Verification items for the finished model (mm, model axes). A direction names the side the tool comes from. Coordinates: 2 decimals unless noted, no trailing zeros. Write each loop counter-clockwise with the first axis right and the second up, starting at its lowest first coordinate (ties: lowest second). Pieces come first, ordered by that corner, then holes. Notation, with made-up numbers: (4.25, -14) - (48.25, -14) arc R22 cw to (48.25, 11) - close; hole circle Ø8 at (47, 0.25). An arc over 180 degrees is marked (long way). Use one line per item in the form item = value. Start each with the question number.
(1) Sectioned sample at B-B (y = -6). Record the cut outline in (x, z) (3 decimals), and give its area (3 significant figures).
(2) Mould release check, pull along Z, two halves, no side actions. Record for faces 1 (the cylindrical face through (-1.57, -12.4, 2.75)), 2 (the flat face through (-1.57, -1.99, 78.3)), 3 (the cylindrical face through (-1.565, -37.718, -5.774)): released by +Z, released by -Z, zero draft, split by the parting line, or undercut.
(3) Gauge pin test, flat end, axial feed: pin 1 Ø1.5 at (x, z) = (-2.5, 69) entering from +Y. Record the tip position at first contact, or that the pin passes through.
(4) Material ranges on line 1 (Y direction, x = -1.25, z = 31.75) (3 decimals); line 2 (Y direction, x = -1.85, z = 2) (3 decimals); line 3 (Y direction, x = -1.85, z = 0), recorded low to high. Write a range as [from, to].
(5) Sectioned sample at C-C (x = -2.4). Count the separate pieces of the cut face and the enclosed holes in it, and give its area (3 significant figures).
(6) Tool access check on faces 4 (the flat face through (-1.565, -38.704, 43.485)), 5 (the cylindrical face through (-1.57, 35.54, 2.3)), 6 (the cylindrical face through (-1.57, 29.59, 41.58)). Record the directions out of +Z, -Z, +X, -X, +Y, -Y that give a thin tool (end or side, any length) a straight path to the whole face; none if there is none.
(7) Sectioned sample at D-D (y = 55). Record the cut outline in (x, z) (3 decimals).
(8) Sectioned sample at A-A (z = 31.5). Record the cut outline in (x, y) (3 decimals), and give its area (3 significant figures).
from build123d import *

# Parameters (mm, degrees)
SKETCH1_W          = 101.6
SKETCH1_H          = 82.55
SKETCH1_R          = 12.7
BASE_FLANGE1_DEPTH = 3.175
SKETCH6_R          = 2.286
CUT_EXTRUDE1_DEPTH = 66.531261624
SKETCH7_R          = 3.175
TAB1_DEPTH         = 3.175
FILLET1_R          = 25.4


# Sheet-metal steps are written as plain solids
with BuildPart() as part:
    # Sketch1 → Base-Flange1 (new body)
    with BuildSketch(Plane(origin=(0, 0, 0), x_dir=(0, 0, -1), z_dir=(1, 0, 0))):
        Rectangle(SKETCH1_W, SKETCH1_H)
        Circle(SKETCH1_R, mode=Mode.SUBTRACT)
    extrude(amount=-BASE_FLANGE1_DEPTH)

    # Sketch6 → Cut-Extrude1 (cut, through all)
    with BuildSketch(Plane(origin=(0, 0, 0), x_dir=(0, 0, -1), z_dir=(1, 0, 0))):
        with BuildLine():
            Line((-50.8, 0), (-50.8, -41.275))
            Line((-50.8, -41.275), (-2, -41.275))
            add(Edge.make_bspline(
                [(-50.8, 0), (-49.405200746, -20.6375), (-31.743734825, -41.275), (-2, -41.275)],
                knots=[0.5, 0.5, 0.5, 0.5, 1, 1, 1, 1], degree=3))
        make_face()
        with BuildLine():
            ThreePointArc((8.260015314, -30.445283168), (5.45906631, -38.06667919), (-2, -41.275))
            Line((-2, -41.275), (50.8, -41.275))
            Line((50.8, -41.275), (50.8, 41.275))
            Line((50.8, 41.275), (-2, 41.275))
            ThreePointArc((-2, 41.275), (5.45906631, 38.06667919), (8.260015314, 30.445283168))
            ThreePointArc((8.260015314, 30.445283168), (9.58920866, 20.855850918), (14.409845519, 12.460291013))
            ThreePointArc((14.409845519, 12.460291013), (19.05, 0), (14.409845519, -12.460291013))
            ThreePointArc((14.409845519, -12.460291013), (9.58920866, -20.855850918), (8.260015314, -30.445283168))
        make_face()
        with BuildLine():
            Line((-50.8, 41.275), (-50.8, 5.257542394))
            add(Edge.make_bspline(
                [(-2, 41.275), (-34.31608403, 41.275), (-49.514685749, 24.001471649), (-50.8, 5.257542394)],
                knots=[0, 0, 0, 0, 0.457437737, 0.457437737, 0.457437737, 0.457437737], degree=3))
            Line((-2, 41.275), (-50.8, 41.275))
        make_face()
        with Locations((-38.862, 0)):
            Circle(SKETCH6_R)
        with Locations((-2, -33.274)):
            Circle(SKETCH6_R)
        with Locations((-2, 33.274)):
            Circle(SKETCH6_R)
    extrude(amount=-CUT_EXTRUDE1_DEPTH, mode=Mode.SUBTRACT)

    # Sketch7 → Tab1 (add)
    # profile 1 of 3: a face of its own
    with BuildSketch(Plane(origin=(0, 0, 0), x_dir=(0, 0, -1), z_dir=(1, 0, 0))):
        with BuildLine():
            Line((-94.917552756, 29.770648167), (-40.208700014, 28.33804644))
            add(Edge.make_bspline(
                [(-40.208700014, 28.33804644), (-46.786875633, 21.92230562), (-50.218303551, 13.740508394), (-50.8, 5.257542394)],
                knots=[0.250414508, 0.250414508, 0.250414508, 0.250414508, 0.457437737, 0.457437737, 0.457437737, 0.457437737], degree=3))
            Line((-50.8, 5.257542394), (-50.8, 0))
            add(Edge.make_bspline(
                [(-50.8, 0), (-50.523888569, -4.085354674), (-49.610330365, -8.170709348), (-48.091785573, -12.095969996)],
                knots=[0.5, 0.5, 0.5, 0.5, 0.598978914, 0.598978914, 0.598978914, 0.598978914], degree=3))
            Line((-48.091785573, -12.095969996), (-99.279769136, 5.031289719))
            ThreePointArc((-99.279769136, 5.031289719), (-107.757058463, 19.280331996), (-94.917552756, 29.770648167))
        make_face()
        with Locations((-95.25, 17.07500014)):
            Circle(SKETCH7_R, mode=Mode.SUBTRACT)
    # profile 2 of 3: a face of its own
    with BuildSketch(Plane(origin=(0, 0, 0), x_dir=(0, 0, -1), z_dir=(1, 0, 0))):
        with BuildLine():
            Line((-44.14895929, -41.701216903), (-40.415374595, -24.860104669))
            add(Edge.make_bspline(
                [(-40.415374595, -24.860104669), (-33.280436064, -33.135041664), (-22.659787261, -39.285311117), (-9.047775931, -40.872784018)],
                knots=[0.713798262, 0.713798262, 0.713798262, 0.713798262, 0.959139114, 0.959139114, 0.959139114, 0.959139114], degree=3))
            Line((-9.047775931, -40.872784018), (-23.170004363, -53.813422177))
            ThreePointArc((-23.170004363, -53.813422177), (-38.1, -55.448522628), (-44.14895929, -41.701216903))
        make_face()
        with Locations((-31.75, -44.45)):
            Circle(SKETCH7_R, mode=Mode.SUBTRACT)
    # profile 3 of 3: a face of its own
    with BuildSketch(Plane(origin=(0, 0, 0), x_dir=(0, 0, -1), z_dir=(1, 0, 0))):
        with BuildLine():
            Line((7.937016423, 63.610827001), (8.211666218, 32.13907772))
            ThreePointArc((8.211666218, 32.13907772), (4.850970786, 38.657664415), (-2, 41.275))
            add(Edge.make_bspline(
                [(-2, 41.275), (-10.740165269, 41.275), (-18.228222741, 40.011477764), (-24.527562549, 37.79707419)],
                knots=[0, 0, 0, 0, 0.123718004, 0.123718004, 0.123718004, 0.123718004], degree=3))
            Line((-24.527562549, 37.79707419), (-17.057975033, 66.679826051))
            ThreePointArc((-17.057975033, 66.679826051), (-3.214759339, 76.105336126), (7.937016423, 63.610827001))
        make_face()
        with Locations((-4.7625, 63.5)):
            Circle(SKETCH7_R, mode=Mode.SUBTRACT)
    extrude(amount=-TAB1_DEPTH)

    # Fillet1
    # the kernel refuses this fillet: 25.4 mm, written as the material it adds along each edge
    with BuildSketch(Plane(origin=(0, -12.095969996, 48.091785573), x_dir=(0, -0.8940853076070706, -0.44789670987982283), z_dir=(-1, 0, 0))) as fillet1_piece_1:
        with BuildLine():
            CenterArc((10.606420456, 25.28678712), FILLET1_R, 225.10881891, 39.479525683)
            Line((-7.319947942, 7.29219582), (-7.67847531, 6.932303994))
            Line((-7.67847531, 6.932303994), (-0.358527368, -0.359891826))
            Line((-0.358527368, -0.359891826), (0.04832888, -0.505695876))
            ThreePointArc((0.04832888, -0.505695876), (4.105397819, -0.313189565), (8.163015374, -0.505735742))
            Line((8.163015374, -0.505735742), (8.210925278, 0))
        make_face()
    extrude(amount=3.175)
    with BuildSketch(Plane(origin=(0, -24.860104669, 40.415374595), x_dir=(0, 0.8184198405618281, 0.5746207136666339), z_dir=(-1, 0, 0))) as fillet1_piece_2:
        with BuildLine():
            CenterArc((11.311656293, -25.273029086), FILLET1_R, 95.731310995, 41.841763873)
            Line((-7.437058628, -8.136935925), (-7.812032926, -7.794214062))
            Line((-7.812032926, -7.794214062), (-0.374974298, 0.342721863))
            Line((-0.374974298, 0.342721863), (0.050418969, 0.505491768))
            ThreePointArc((0.050418969, 0.505491768), (4.387605763, 0.289082367), (8.724392403, 0.505460582))
            Line((8.724392403, 0.505460582), (8.775123067, 0))
        make_face()
    extrude(amount=3.175)
    with BuildSketch(Plane(origin=(0, -40.872784018, 9.047775931), x_dir=(0, -0.04853483979472319, -0.9988214902204), z_dir=(-1, 0, 0))) as fillet1_piece_3:
        with BuildLine():
            CenterArc((10.770038636, 25.222537483), FILLET1_R, 224.718065589, 38.505093781)
            Line((-7.27863381, 7.350620325), (-9.083501055, 5.563428609))
            Line((-9.083501055, 5.563428609), (-1.804867245, -1.787191716))
            Line((-1.804867245, -1.787191716), (0.171432812, -2.534208119))
            ThreePointArc((0.171432812, -2.534208119), (6.935713053, -2.477327294), (7.473046138, -2.522253748))
            Line((7.473046138, -2.522253748), (7.772772728, 0))
        make_face()
    extrude(amount=3.175)
    with BuildSketch(Plane(origin=(0, 28.33804644, 40.208700014), x_dir=(0, 0.6273452084860717, -0.7787412852735929), z_dir=(-1, 0, 0))) as fillet1_piece_4:
        with BuildLine():
            CenterArc((9.459006839, -25.293729314), FILLET1_R, 95.242990238, 35.111537056)
            Line((-6.987881866, -5.937597161), (-7.31681964, -5.550474518))
            Line((-7.31681964, -5.550474518), (-0.328937774, 0.387122643))
            Line((-0.328937774, 0.387122643), (0.048065336, 0.505720994))
            ThreePointArc((0.048065336, 0.505720994), (3.568700205, 0.341549606), (7.091539297, 0.505874586))
            Line((7.091539297, 0.505874586), (7.137960229, 0))
        make_face()
    extrude(amount=3.175)
    with BuildSketch(Plane(origin=(0, 37.79707419, 24.527562549), x_dir=(0, -0.42252064373268267, 0.9063533006613478), z_dir=(-1, 0, 0))) as fillet1_piece_5:
        with BuildLine():
            CenterArc((12.096936965, 25.25943543), FILLET1_R, 219.493828852, 44.475589611)
            Line((-7.504067493, 9.105159703), (-7.896087582, 8.782074189))
            Line((-7.896087582, 8.782074189), (-0.392020089, -0.323085515))
            Line((-0.392020089, -0.323085515), (0.049799336, -0.505553188))
            ThreePointArc((0.049799336, -0.505553188), (4.714693558, -0.268029159), (9.375061322, -0.505188709))
            Line((9.375061322, -0.505188709), (9.428431432, 0))
        make_face()
    extrude(amount=3.175)
    with BuildSketch(Plane(origin=(0, 32.13907772, -8.211666218), x_dir=(0, -0.9961860509350137, -0.08725452379391116), z_dir=(-1, 0, 0))) as fillet1_piece_6:
        with BuildLine():
            CenterArc((1.089917285, -25.392853706), FILLET1_R, 91.359162517, 3.146518864)
            Line((-0.905454606, -0.071351164), (-0.945362044, 0.435078887))
            Line((-0.945362044, 0.435078887), (-0.039907438, 0.506430051))
            Line((-0.039907438, 0.506430051), (0.012049575, 0.507857074))
            ThreePointArc((0.012049575, 0.507857074), (0.243719262, 0.505109127), (0.47538895, 0.507857074))
            Line((0.47538895, 0.507857074), (0.487438525, 0))
        make_face()
    extrude(amount=3.175)


solid = part.part
Answers below:
q1.outline = (-3.175, -18.08) - (0, -18.08) - (0, -11.193) - (-3.175, -11.193) - close; (-3.175, 11.193) - (0, 11.193) - (0, 66.311) - (-3.175, 66.311) - close
q1.area = 197 mm2
q2.face_1 = undercut
q2.face_2 = released by +Z
q2.face_3 = released by -Z
q3.pin_1 = 29.11
q4.line_1 = [-57.15, -47.625], [-41.275, 34.666]
q4.line_2 = [-41.31, -35.56], [-30.988, -12.542], [12.542, 30.988], [35.56, 61.935], [65.065, 75.896]
q4.line_3 = [-41.08, -34.38], [-32.17, -12.7], [12.7, 32.17], [34.38, 75.27]
q5.separate_pieces = 1
q5.enclosed_holes = 7
q5.area = 7,080 mm2
q6.face_4 = +Z, +X, -X
q6.face_5 = +X, -X
q6.face_6 = +X, -X, +Y
q7.outline = (-3.175, -8.012) - (0, -8.012) - (0, 20.079) - (-3.175, 20.079) - close
q8.outline = (-3.175, -57.148) - (0, -57.148) - (0, -47.615) - (-3.175, -47.615) - close; (-3.175, -41.285) - (0, -41.285) - (0, 34.841) - (-3.175, 34.841) - close
q8.area = 272 mm2
